Design review of the part built by this model. Coordinates are the model's own, in mm. A direction names the side the tool comes from. Give positions to 0.01 mm unless a question says otherwise; leave off trailing zeros. Write each loop counter-clockwise with the first axis right and the second up, starting at its lowest first coordinate (ties: lowest second). Pieces come first, ordered by that corner, then holes. Notation, with made-up numbers: (-16, 11) -> (-10, 11) arc R20 ccw to (-10, 32) -> close; hole circle Ø8 at (-39.5, 55). An arc over 180 degrees is marked (long way). Answer as a JSON object with one key per item and string values.
```python
from build123d import *

# Parameters (mm, degrees)
RESSALTO_EXTRUS_O1_DEPTH = 5
ESBO_O2_R                = 1.5
CORTE_EXTRUS_O1_DEPTH    = 5
ESBO_O3_R                = 1.5
CORTE_EXTRUS_O2_DEPTH    = 6
ESBO_O6_W                = 3
ESBO_O6_H                = 25
ESBO_O6_W_2              = 25
ESBO_O6_H_2              = 3
CORTE_EXTRUS_O4_DEPTH    = 6


with BuildPart() as part:
    # Esboço1 → Ressalto-extrusão1 (new body)
    with BuildSketch(Plane.XY):
        with BuildLine():
            Line((-49.217119449, -36.393854661), (60.782880551, -36.393854661))
            ThreePointArc((60.782880551, -36.393854661), (67.853948363, -33.464922473), (70.782880551, -26.393854661))
            Line((70.782880551, -26.393854661), (70.782880551, 118.606145339))
            ThreePointArc((70.782880551, 118.606145339), (67.853948363, 125.67721315), (60.782880551, 128.606145339))
            Line((60.782880551, 128.606145339), (-49.217119449, 128.606145339))
            ThreePointArc((-49.217119449, 128.606145339), (-56.288187261, 125.67721315), (-59.217119449, 118.606145339))
            Line((-59.217119449, 118.606145339), (-59.217119449, -26.393854661))
            ThreePointArc((-59.217119449, -26.393854661), (-56.288187261, -33.464922473), (-49.217119449, -36.393854661))
        make_face()
    extrude(amount=RESSALTO_EXTRUS_O1_DEPTH)

    # Esboço2 → Corte-extrusão1 (cut)
    with BuildSketch(Plane(origin=(0, 0, 0), x_dir=(-1, 0, 0), z_dir=(0, 0, -1))):
        with Locations((33.717119449, -15.893854661)):
            Circle(ESBO_O2_R)
        with Locations((33.717119449, 108.106145339)):
            Circle(ESBO_O2_R)
        with Locations((-45.282880551, -15.893854661)):
            Circle(ESBO_O2_R)
        with Locations((-45.282880551, 108.106145339)):
            Circle(ESBO_O2_R)
    extrude(amount=-CORTE_EXTRUS_O1_DEPTH, mode=Mode.SUBTRACT)

    # Esboço3 → Corte-extrusão2 (cut, through all)
    with BuildSketch(Plane(origin=(0, 0, 0), x_dir=(-1, 0, 0), z_dir=(0, 0, -1))):
        with Locations((49.217119449, 118.606145339)):
            Circle(ESBO_O3_R)
        with Locations((49.217119449, 76.556145339)):
            Circle(ESBO_O3_R)
    extrude(amount=-CORTE_EXTRUS_O2_DEPTH, mode=Mode.SUBTRACT)

    # Esboço6 → Corte-extrusão4 (cut, through all)
    with BuildSketch(Plane(origin=(0, 0, 0), x_dir=(-1, 0, 0), z_dir=(0, 0, -1))):
        with Locations((-67.282880551, -13.893854661)):
            Rectangle(ESBO_O6_W, ESBO_O6_H)
        with Locations((-67.282880551, 41.106145339)):
            Rectangle(ESBO_O6_W, ESBO_O6_H)
        with Locations((-48.282880551, 40.106145339)):
            Rectangle(ESBO_O6_W_2, ESBO_O6_H_2)
        with Locations((36.717119449, 40.106145339)):
            Rectangle(ESBO_O6_W_2, ESBO_O6_H_2)
        with Locations((55.717119449, 38.28693606)):
            Rectangle(ESBO_O6_W, ESBO_O6_H)
        with Locations((55.717119449, -13.893854661)):
            Rectangle(ESBO_O6_W, ESBO_O6_H)
        with Locations((-5.782880551, 40.106145339)):
            Rectangle(ESBO_O6_W_2, ESBO_O6_H_2)
    extrude(amount=-CORTE_EXTRUS_O4_DEPTH, mode=Mode.SUBTRACT)


solid = part.part
```
(1) We need section C-C, the plane z = 1.6. Give the number of separate pieces and of enclosed holes in the cut face, then the cut area to 3 significant figures.
Here are the results:
{"separate pieces": "1", "enclosed holes": "13", "area": "20,800 mm²"}
(2) The part is to be moulded in two halves that separate along X. For faces 1 (the cylindrical face through (67.93, 125.6, 2.46)), 2 (the flat face through (5, -36.394, 2)), 3 (the flat face through (68.783, -14, 2)), say which applies: +X half, -X half, draft (parallel to the pull), parting line (faces both ways), or undercut.
Here are the results:
{"face 1": "+X half", "face 2": "draft", "face 3": "undercut"}
(3) For faces 4 (the flat face through (68.783, 41, 2)), 5 (the cylindrical face through (67.78, -33.54, 2.46)), list the 3-axis set-ups (+Z, -Z, +X, -X, +Y, -Y) from which the entire face can be reached by the end or side of a thin tool; tool diameter is ignored.
Here are the results:
{"face 4": "+Z, -Z", "face 5": "+Z, -Z, +X, -Y"}
(4) For line 1 along X through (y, z) = (35, 4.55); line 2 along X through (y, z) = (40, 4.55); line 3 along Y through (x, z) = (4, 2.25), list the stretches that pass through material, from the lowest coordinate up.
Here are the results:
{"line 1": "x = -59.22 to -57.22, -54.22 to 65.78, 68.78 to 70.78", "line 2": "x = -59.22 to -57.22, -54.22 to -49.22, -24.22 to -6.72, 18.28 to 35.78, 60.78 to 65.78, 68.78 to 70.78", "line 3": "y = -36.39 to 38.61, 41.61 to 128.61"}
(5) We need section B-B, the plane y = 44.5. State the section outline as (x, z) points.
Here are the results:
{"outline": "(-59.22, 0) -> (-57.22, 0) -> (-57.22, 5) -> (-59.22, 5) -> close; (-54.22, 0) -> (65.78, 0) -> (65.78, 5) -> (-54.22, 5) -> close; (68.78, 0) -> (70.78, 0) -> (70.78, 5) -> (68.78, 5) -> close"}
(6) Clearance check with flat-ended pins moving along their axes: pin 1 (2.5 mm diameter, centred on x = -49.22, y = 76.56, fed in from +Z); pin 2 (0.9 mm diameter, centred on x = 67, z = 1.5, fed in from +Y); pin 3 (2.5 mm diameter, centred on x = 67, z = 2, fed in from -Y); pin 4 (1.5 mm diameter, centred on x = -56, z = 3.5, fed in from -Y). State where each tip first meets the part, or that it passes through.
Here are the results:
{"pin 1": "passes through", "pin 2": "stops at y = 126.78", "pin 3": "stops at y = -35.07", "pin 4": "stops at y = -34.37"}
(7) We need section A-A, the plane x = -41. State the section outline as (y, z) points, then the cut area to 3 significant figures.
Here are the results:
{"outline": "(-36.39, 0) -> (38.61, 0) -> (38.61, 5) -> (-36.39, 5) -> close; (41.61, 0) -> (128.61, 0) -> (128.61, 5) -> (41.61, 5) -> close", "area": "810 mm²"}
